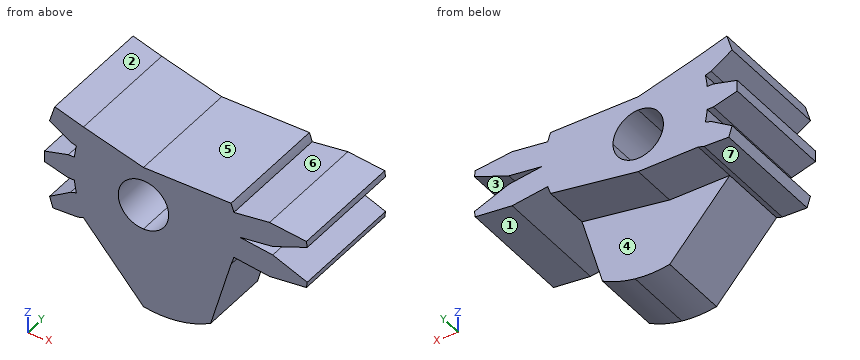
from build123d import *

# Parameters (mm, degrees)
BOSS_EXTRUDE1_DEPTH = 9.7
BOSS_EXTRUDE2_DEPTH = 5.8
CUT_EXTRUDE1_DEPTH  = 15.880557968
BOSS_EXTRUDE9_REACH = 16.881
BOSS_EXTRUDE8_START = -9.7
BOSS_EXTRUDE8_DEPTH = 9.7
BOSS_EXTRUDE5_DEPTH = 5.8
CUT_EXTRUDE2_DEPTH  = 9.7


# Read off the part's stored shape, not the designer's step: Boss-Extrude8
with BuildPart() as part:
    # Sketch1 → Boss-Extrude1 (new body)
    with BuildSketch(Plane(origin=(0, 0, 0), x_dir=(1, 0, 0), z_dir=(0, 1, 0))):
        Polygon((6.15, 2.65), (6.15, -2.65), (-1.15, -2.65), (-6.15, -4.038578044), (-6.15, 3.861421956), (-1.15, 3.861421956), align=None)
    extrude(amount=BOSS_EXTRUDE1_DEPTH)

    # Sketch2 → Boss-Extrude2 (add)
    with BuildSketch(Plane.XZ):
        Polygon((-6.15, -3.861421956), (-1.15, -9.461421956), (-1.15, -3.861421956), align=None)
        Polygon((-1.15, -3.861421956), (-1.15, -9.461421956), (4.45, -8.532111962), (4.45, -2.932111962), align=None)
        Polygon((4.45, -2.932111962), (4.45, -8.532111962), (6.15, -2.65), align=None)
    extrude(amount=-BOSS_EXTRUDE2_DEPTH)

    # Sketch3 → Cut-Extrude1 (cut, through all)
    with BuildSketch(Plane(origin=(0, 9.7, 0), x_dir=(1, 0, 0), z_dir=(0, 1, 0))):
        with BuildLine():
            ThreePointArc((0.95, 0.605710978), (0.33492424, 2.090635219), (-1.15, 2.705710978))
            Line((-1.15, 2.705710978), (-1.15, -1.494289022))
            ThreePointArc((-1.15, -1.494289022), (0.33492424, -0.879213262), (0.95, 0.605710978))
        make_face()
        with BuildLine():
            Line((-1.15, -1.494289022), (-1.15, 2.705710978))
            ThreePointArc((-1.15, 2.705710978), (-3.25, 0.605710978), (-1.15, -1.494289022))
        make_face()
    extrude(amount=-CUT_EXTRUDE1_DEPTH, mode=Mode.SUBTRACT)

    # Boss-Extrude9: up to this face of the body (flat: up to its plane)
    boss_extrude9_end = Plane(part.part.faces().sort_by_distance((0.174384558, 0, -2.694350329))[0])
    # Sketch4 → Boss-Extrude9 (add, up to the picked face)
    with BuildSketch(Plane(origin=(0, 9.7, 0), x_dir=(1, 0, 0), z_dir=(0, 1, 0)), mode=Mode.PRIVATE) as boss_extrude9_sk1:
        with BuildLine():
            Line((12.596453684, 0.767826071), (12.330020735, 2.75))
            Line((12.330020735, 2.75), (6.383498949, 1.950701151))
            ThreePointArc((6.383498949, 1.950701151), (6.27561663, 2.303311358), (6.15, 2.65))
            Line((6.15, 2.65), (6.15, -2.65))
            ThreePointArc((6.15, -2.65), (6.27561663, -2.303311358), (6.383498949, -1.950701151))
            Line((6.383498949, -1.950701151), (12.330020735, -2.75))
            Line((12.330020735, -2.75), (12.596453684, -0.767826071))
            Line((12.596453684, -0.767826071), (6.884079059, 0))
            Line((6.884079059, 0), (12.596453684, 0.767826071))
        make_face()
    boss_extrude9_tool1 = split(extrude(boss_extrude9_sk1.sketch, amount=-BOSS_EXTRUDE9_REACH, mode=Mode.PRIVATE), bisect_by=boss_extrude9_end, keep=Keep.BOTH, mode=Mode.PRIVATE)
    add(boss_extrude9_tool1.solids().sort_by(Axis((6.19524, 9.7, -2.276473), (0, -1, 0)))[0])

    # Boss-Extrude8 outline → Boss-Extrude8 (add)
    with BuildSketch(Plane(origin=(0, 9.7, 0), x_dir=(1, 0, 0), z_dir=(0, 1, 0)).offset(BOSS_EXTRUDE8_START)):
        with BuildLine():
            Line((-7.223773577, -2.277754847), (-8.969746456, -3.387643024))
            Line((-8.969746456, -3.387643024), (-8.537608436, -4.779743311))
            Line((-8.537608436, -4.779743311), (-6.15, -4.038578044))
            Line((-6.15, -4.038578044), (-6.15, 3.861421956))
            Line((-6.15, 3.861421956), (-6.627521687, 4.00965501))
            Line((-6.627521687, 4.00965501), (-8.696484144, 4.090781022))
            Line((-8.696484144, 4.090781022), (-8.971664943, 3.204306677))
            Line((-8.971664943, 3.204306677), (-7.220453901, 2.099568261))
            Line((-7.220453901, 2.099568261), (-6.742932214, 1.951335207))
            ThreePointArc((-6.742932214, 1.951335207), (-6.835256527, 1.433422288), (-6.900626431, 0.911421956))
            Line((-6.900626431, 0.911421956), (-7.405143495, 0.911421956))
            Line((-7.405143495, 0.911421956), (-9.400626431, 0.373036291))
            Line((-9.400626431, 0.373036291), (-9.400626431, -0.556661548))
            Line((-9.400626431, -0.556661548), (-7.401686619, -1.088575255))
            Line((-7.401686619, -1.088575255), (-6.900626431, -1.088578044))
            ThreePointArc((-6.900626431, -1.088578044), (-6.835256527, -1.610578376), (-6.742932214, -2.128491295))
            Line((-6.742932214, -2.128491295), (-7.223773577, -2.277754847))
        make_face()
    extrude(amount=BOSS_EXTRUDE8_DEPTH)

    # Sketch8 → Boss-Extrude5 (add)
    with BuildSketch(Plane(origin=(0, 5.8, 0), x_dir=(1, 0, 0), z_dir=(0, 1, 0))):
        with BuildLine():
            ThreePointArc((1.731854671, 9.490021268), (0.289677429, 9.601670434), (-1.15, 9.461421956))
            Line((-1.15, 9.461421956), (1.65, 8.996766959))
            Line((1.65, 8.996766959), (1.731854671, 9.490021268))
        make_face()
        with BuildLine():
            Line((1.731854671, 9.490021268), (1.65, 8.996766959))
            Line((1.65, 8.996766959), (4.45, 8.532111962))
            ThreePointArc((4.45, 8.532111962), (3.132791885, 9.12986067), (1.731854671, 9.490021268))
        make_face()
    extrude(amount=-BOSS_EXTRUDE5_DEPTH)

    # Sketch5 → Cut-Extrude2 (cut)
    with BuildSketch(Plane(origin=(0, 9.7, 0), x_dir=(1, 0, 0), z_dir=(0, 1, 0))):
        Polygon((9.623192791, 0.368176647), (12.596453684, 0.767826071), (12.496541328, 1.511141295), align=None)
        Polygon((9.356759842, 2.350350576), (12.429933091, 2.006684777), (12.330020735, 2.75), align=None)
        Polygon((12.429933091, -2.006684777), (12.330020735, -2.75), (9.356759842, -2.350350576), align=None)
        Polygon((12.596453684, -0.767826071), (12.496541328, -1.511141295), (9.623192791, -0.368176647), align=None)
    extrude(amount=-CUT_EXTRUDE2_DEPTH, mode=Mode.SUBTRACT)


solid = part.part
Build history of the part. All positions in model axes, mm. Face numbers are marked on the shaded views. A direction names the side the tool comes from. Round coordinates to 2 decimals unless told otherwise and drop trailing zeros. Write each loop counter-clockwise with the first axis right and the second up, starting at its lowest first coordinate (ties: lowest second). Pieces come first, ordered by that corner, then holes. Notation, with made-up numbers: M 83,2 L 131,2 A18 cw 131,30 Z; hole C 89.25,84.25 d6. An arc over 180 degrees is marked long. Answer in a Markdown table with one row per item.
1. Flat gauge pins, fed straight in: P1, Ø3, axis at x = -0.5, z = 1, coming from the +Y side; P2, Ø4, axis at x = -2.5, y = 8.5, coming from the +Z side; P3, Ø1.9, axis at x = -4, y = 8.5, coming from the -Z side; P4, Ø2, axis at x = -1.5, z = -8, coming from the +Y side. Where does each tip first touch, or does it go through?
Geometry check:
| item | result |
|---|---|
| P1 | y = 9.7 |
| P2 | z = 3.58 |
| P3 | z = -3.86 |
| P4 | y = 5.8 |
2. Saw through at B-B (x = -4.25). List the corners of the cut face in (y, z), and give its area (3 significant figures).
Geometry check:
| item | result |
|---|---|
| outline | M 0,-5.99 L 5.8,-5.99 L 5.8,-3.86 L 9.7,-3.86 L 9.7,3.51 L 0,3.51 Z |
| area | 83.9 mm2 |
3. Saw through at A-A (x = 8). List the corners of the cut face in (y, z).
Geometry check:
| item | result |
|---|---|
| outline | M 0,-2.17 L 9.7,-2.17 L 9.7,-0.15 L 0,-0.15 Z; M 0,0.15 L 9.7,0.15 L 9.7,2.17 L 0,2.17 Z |
4. Probe L1, parallel to Y at x = -2, z = -5.5; L2, parallel to Z at x = -7.5, y = 8; L3, parallel to Z at x = 9.75, y = 6.75. List the from-to ranges inside material, lowest first. Write a range as [from, to].
Geometry check:
| item | result |
|---|---|
| L1 | [0, 5.8] |
| L2 | [-4.04, -2.28], [-0.89, 1.06], [2.45, 4.46] |
| L3 | [-2.31, -0.42], [0.42, 2.31] |
5. Which spindle directions (+Z, -Z, +X, -X, +Y, -Y) get a long thin tool onto all of the face, cutting with end or side? Do the marked faces 4, 5, 6 and 7. Say none if no direction does.
Geometry check:
| item | result |
|---|---|
| face 4 | -Z, +X, +Y |
| face 5 | +Z, +X, +Y, -Y |
| face 6 | +Z, +Y, -Y |
| face 7 | -Z, +Y, -Y |
6. Mould opens along Z. For the marked faces 1, 2 and 3 say: +Z half, -Z half, draft (parallel to the pull), parting line (faces both ways), or undercut.
Geometry check:
| item | result |
|---|---|
| face 1 | -Z half |
| face 2 | +Z half |
| face 3 | undercut |
